from build123d import *

# Parameters (mm, degrees)
F0_R         = 16.5608
F0_R_2       = 11.4808
F1_DEPTH     = 198.4502
F4_DEPTH     = 82.804
F5_T4_DEPTH  = 43.6852975665
F5_S5_R      = 16.5608
F5_T6_DEPTH  = 27
F5_S7_R      = 11.4808
F5_T8_DEPTH  = 27
F5_T12_DEPTH = 43.6852975665
F5_S13_R     = 16.5608
F5_T14_DEPTH = 27
F5_S15_R     = 11.4808
F5_T16_DEPTH = 27
F5_T20_DEPTH = 43.6852975665
F5_S21_R     = 16.5608
F5_T22_DEPTH = 27
F5_S23_R     = 11.4808
F5_T24_DEPTH = 27
F5_T28_DEPTH = 43.6852975665
F5_S29_R     = 16.5608
F5_T30_DEPTH = 27
F5_S31_R     = 11.4808
F5_T32_DEPTH = 27


# Not quite as in the source:
# - a fillet or chamfer that OpenCascade refuses, or shapes differently, is made with other operations: its cross-section is extruded or revolved along the edge and cut away or added


with BuildPart() as f1:
    # F0 (on Front) → F1 (new body)
    with BuildSketch(Plane.XZ):
        Circle(F0_R)
        Circle(F0_R_2, mode=Mode.SUBTRACT)
    extrude(amount=F1_DEPTH)

    # F3 (on offset) → F4 (cut)
    with BuildSketch(Plane(origin=(0, -96.0882, 0), x_dir=(-1, 0, 0), z_dir=(0, 1, 0))):
        with BuildLine():
            Line((7.9590822086, -8.2741633436), (16.5608, 0))
            ThreePointArc((16.5608, 0), (11.7102539819, 11.7102539819), (0, 16.5608))
            Line((0, 16.5608), (-8.2741633436, 7.9590822086))
            Line((-8.2741633436, 7.9590822086), (7.9590822086, -8.2741633436))
        make_face()
    extrude(amount=-F4_DEPTH, mode=Mode.SUBTRACT)

    # F5: fillet of radius 6.35 on 4 edges, made by hand


with BuildPart() as f5_tool2:
    # F5_s3 → F5_t4 (new body)
    with BuildSketch(Plane(origin=(-19.2795314418, 0, 20.0427622378), x_dir=(0, 1, 0), z_dir=(0.6932515337, 0, -0.7206957132))):
        with BuildLine():
            ThreePointArc((-102.4382, 11.4808), (-97.9480719395, 9.6209280605), (-96.0882, 5.1308))
            Line((-96.0882, 5.1308), (-96.0882, 11.4808))
            Line((-96.0882, 11.4808), (-102.4382, 11.4808))
        make_face()
    extrude(amount=F5_T4_DEPTH)

    # F5_s5 → F5_t6 (intersect, symmetric)
    with BuildSketch(Plane.XZ.offset(99.3)):
        Circle(F5_S5_R)
    extrude(amount=F5_T6_DEPTH, both=True, mode=Mode.INTERSECT)

    # F5_s7 → F5_t8 (cut, symmetric)
    with BuildSketch(Plane.XZ.offset(99.3)):
        Circle(F5_S7_R)
    extrude(amount=F5_T8_DEPTH, both=True, mode=Mode.SUBTRACT)


with BuildPart() as f1_1:
    add(f1.part)

    # F5_t1: union F5_tool2
    add(f5_tool2.part)


with BuildPart() as f5_tool10:
    # F5_s11 → F5_t12 (new body)
    with BuildSketch(Plane(origin=(11.4410444464, 0, -11.0053680982), x_dir=(0, 1, 0), z_dir=(-0.7206957132, 0, 0.6932515337))):
        with BuildLine():
            ThreePointArc((-102.4382, 11.4808), (-97.9480719395, 9.6209280605), (-96.0882, 5.1308))
            Line((-96.0882, 5.1308), (-96.0882, 11.4808))
            Line((-96.0882, 11.4808), (-102.4382, 11.4808))
        make_face()
    extrude(amount=F5_T12_DEPTH)

    # F5_s13 → F5_t14 (intersect, symmetric)
    with BuildSketch(Plane.XZ.offset(99.3)):
        Circle(F5_S13_R)
    extrude(amount=F5_T14_DEPTH, both=True, mode=Mode.INTERSECT)

    # F5_s15 → F5_t16 (cut, symmetric)
    with BuildSketch(Plane.XZ.offset(99.3)):
        Circle(F5_S15_R)
    extrude(amount=F5_T16_DEPTH, both=True, mode=Mode.SUBTRACT)


with BuildPart() as f1_2:
    add(f1_1.part)

    # F5_t9: union F5_tool10
    add(f5_tool10.part)


with BuildPart() as f5_tool18:
    # F5_s19 → F5_t20 (new body)
    with BuildSketch(Plane(origin=(-19.2795314418, 0, 20.0427622378), x_dir=(0, 1, 0), z_dir=(0.6932515337, 0, -0.7206957132))):
        with BuildLine():
            ThreePointArc((-172.5422, 11.4808), (-177.0323280605, 9.6209280605), (-178.8922, 5.1308))
            Line((-178.8922, 5.1308), (-178.8922, 11.4808))
            Line((-178.8922, 11.4808), (-172.5422, 11.4808))
        make_face()
    extrude(amount=F5_T20_DEPTH)

    # F5_s21 → F5_t22 (intersect, symmetric)
    with BuildSketch(Plane.XZ.offset(175.7)):
        Circle(F5_S21_R)
    extrude(amount=F5_T22_DEPTH, both=True, mode=Mode.INTERSECT)

    # F5_s23 → F5_t24 (cut, symmetric)
    with BuildSketch(Plane.XZ.offset(175.7)):
        Circle(F5_S23_R)
    extrude(amount=F5_T24_DEPTH, both=True, mode=Mode.SUBTRACT)


with BuildPart() as f1_3:
    add(f1_2.part)

    # F5_t17: union F5_tool18
    add(f5_tool18.part)


with BuildPart() as f5_tool26:
    # F5_s27 → F5_t28 (new body)
    with BuildSketch(Plane(origin=(11.4410444464, 0, -11.0053680982), x_dir=(0, 1, 0), z_dir=(-0.7206957132, 0, 0.6932515337))):
        with BuildLine():
            ThreePointArc((-178.8922, 5.1308), (-177.0323280605, 9.6209280605), (-172.5422, 11.4808))
            Line((-172.5422, 11.4808), (-178.8922, 11.4808))
            Line((-178.8922, 11.4808), (-178.8922, 5.1308))
        make_face()
    extrude(amount=F5_T28_DEPTH)

    # F5_s29 → F5_t30 (intersect, symmetric)
    with BuildSketch(Plane.XZ.offset(175.7)):
        Circle(F5_S29_R)
    extrude(amount=F5_T30_DEPTH, both=True, mode=Mode.INTERSECT)

    # F5_s31 → F5_t32 (cut, symmetric)
    with BuildSketch(Plane.XZ.offset(175.7)):
        Circle(F5_S31_R)
    extrude(amount=F5_T32_DEPTH, both=True, mode=Mode.SUBTRACT)


with BuildPart() as f1_4:
    add(f1_3.part)

    # F5_t25: union F5_tool26
    add(f5_tool26.part)


solid = f1_4.part
Geometry: final body of the model. Coordinates: model frame, mm. A direction names the side the tool comes from. Give positions to 0.01 mm unless a question says otherwise; leave off trailing zeros. Write each loop counter-clockwise with the first axis right and the second up, starting at its lowest first coordinate (ties: lowest second). Pieces come first, ordered by that corner, then holes.
(1) Mould query, pull axis X, two halves, no side actions, for faces 1 (the flat face through (4.1, -137, 12.3)), 2 (the cylindrical face through (-14.046, -98.853, -0.881)), 3 (the flat face through (-4, 0, -11)). Classes: released by +X, released by -X, zero draft, split by the parting line, or undercut.
(2) Access query for faces 4 (the flat face through (-10, -178.892, 9)), 5 (the flat face through (-4, -198.45, -11)), 6 (the cylindrical face through (-13.99, -176.241, -0.823)), 7 (the cylindrical face through (0.73, -98.85, 14.2)). Directions: +Z, -Z, +X, -X, +Y, -Y. A direction counts if a zero-diameter tool reaches every point of the face in a straight line with its end or side. Return the directions, or none.
(3) Cut plane B-B, the plane z = -13.5. Return loops of the section in (x, y), then the cut area to 3 significant figures.
(4) Ray query, line 1 (Z direction, x = 0, y = -76); line 2 (Y direction, x = -7.5, z = 13.5). Return the intervals inside material, ascending.
(5) First-contact query: P1, Ø6, axis at x = 3.5, y = -28, coming from the -Z side; P2, Ø6, axis at x = -12, y = -118, coming from the -Z side; P3, Ø1.5, axis at y = -129.5, z = -2.5, coming from the -X side. Flat tips, straight axial feed; report the tip coordinate or a pass-through.
(6) Cut plane C-C, the plane y = -132. Return loops of the section in (x, z), then the cut area to 3 significant figures.
(7) Cut plane A-A, the plane y = -40. Return loops of the section in (x, z), then the cut area to 3 significant figures.
Values follow:
1. face 1: released by -X
1. face 2: undercut
1. face 3: zero draft
2. face 4: none
2. face 5: +Z, -Z, +X, -X, -Y
2. face 6: +Z
2. face 7: -X
3. outline: (-9.59, -198.45) - (9.59, -198.45) - (9.59, 0) - (-9.59, 0) - close
3. area: 3,810 mm2
4. line 1: z = -16.56 to -11.48, 11.48 to 16.56
4. line 2: y = -198.45 to -178.89, -96.09 to 0
5. P1: stops at z = -16.55
5. P2: stops at z = -13.9
5. P3: stops at x = -16.47
6. outline: (-16.56, 0) arc R16.56 ccw (long way) to (0, 16.56) - (8.27, 7.96) arc R11.48 cw to (-7.96, -8.27) - close
6. area: 305 mm2
7. outline: circle Ø33.12 at (0, 0); hole circle Ø22.96 at (0, 0)
7. area: 448 mm2
